from build123d import *

# Parameters (mm, degrees)
F0_R     = 2.38125
F1_DEPTH = 6.35


with BuildPart() as f1:
    # F0 (on Top) → F1 (new body)
    with BuildSketch(Plane.XY):
        with BuildLine():
            Line((77.357605, 85.293555), (-62.342395, 85.293555))
            Line((-62.342395, 85.293555), (-62.342395, 40.843555))
            Line((-62.342395, 40.843555), (-46.467395, 40.843555))
            ThreePointArc((-46.467395, 40.843555), (-41.977267, 38.983683), (-40.117395, 34.493555))
            Line((-40.117395, 34.493555), (-40.117395, -48.056445))
            ThreePointArc((-40.117395, -48.056445), (-41.977267, -52.546573), (-46.467395, -54.406445))
            Line((-46.467395, -54.406445), (-62.342395, -54.406445))
            Line((-62.342395, -54.406445), (-62.342395, -98.856445))
            Line((-62.342395, -98.856445), (-11.542395, -98.856445))
            Line((-11.542395, -98.856445), (77.357605, -98.856445))
            Line((77.357605, -98.856445), (77.357605, -54.406445))
            Line((77.357605, -54.406445), (61.482605, -54.406445))
            ThreePointArc((61.482605, -54.406445), (56.992477, -52.546573), (55.132605, -48.056445))
            Line((55.132605, -48.056445), (55.132605, 34.493555))
            ThreePointArc((55.132605, 34.493555), (56.992477, 38.983683), (61.482605, 40.843555))
            Line((61.482605, 40.843555), (77.357605, 40.843555))
            Line((77.357605, 40.843555), (77.357605, 85.293555))
        make_face()
        with Locations((-11.542395, -60.756445)):
            Circle(F0_R, mode=Mode.SUBTRACT)
        with Locations((26.557605, -60.756445)):
            Circle(F0_R, mode=Mode.SUBTRACT)
        with Locations((-40.117395, 45.606055)):
            Circle(F0_R, mode=Mode.SUBTRACT)
        with Locations((-33.767395, 40.843555)):
            Circle(F0_R, mode=Mode.SUBTRACT)
        with Locations((-40.117395, 66.243555)):
            Circle(F0_R, mode=Mode.SUBTRACT)
        with Locations((-40.117395, 80.531055)):
            Circle(F0_R, mode=Mode.SUBTRACT)
        with Locations((48.782605, 40.843555)):
            Circle(F0_R, mode=Mode.SUBTRACT)
        with Locations((55.132605, 45.606055)):
            Circle(F0_R, mode=Mode.SUBTRACT)
        with Locations((55.132605, 66.243555)):
            Circle(F0_R, mode=Mode.SUBTRACT)
        with Locations((55.132605, 80.531055)):
            Circle(F0_R, mode=Mode.SUBTRACT)
    extrude(amount=F1_DEPTH)


solid = f1.part
Model file for the job. Use its own axes, mm. A direction names the side the tool comes from. Give positions to 0.01 mm unless a question says otherwise; leave off trailing zeros. Write each loop counter-clockwise with the first axis right and the second up, starting at its lowest first coordinate (ties: lowest second). Pieces come first, ordered by that corner, then holes. Notation, with made-up numbers: (76.5, 8.25) - (98.5, 8.25) arc R18 cw to (98.5, 17.25) - close; hole circle Ø2 at (30.5, 20). An arc over 180 degrees is marked (long way). Answer as CSV lines item,"result".
1. Band-saw the part on C-C (y = -32.5). Write the cut outline in (x, z), and give its area (3 significant figures).
Responses:
outline,"(-40.12, 0) - (55.13, 0) - (55.13, 6.35) - (-40.12, 6.35) - close"
area,"605 mm2"
2. Drill centre lines: L1, parallel to Y at x = -40, z = 6.25; L2, parallel to Y at x = 54, z = 0.75; L3, parallel to Y at x = 49, z = 3.75. Where is each one in solid material? Low to high. Write a range as [from, to].
Responses:
L1,"y = [-98.86, 43.23], [47.98, 63.87], [68.62, 78.15], [82.91, 85.29]"
L2,"y = [-98.86, 43.51], [47.7, 64.15], [68.34, 78.44], [82.63, 85.29]"
L3,"y = [-98.86, 38.47], [43.21, 85.29]"
3. Two-plate mould, pull along Y, no slides. Class faces 1 (the face through (28.757, -61.668, 3.131)), 2 (the face through (77.358, -77, 3)), 3 (the face through (8, 85.294, 3)): +Y half, -Y half, draft (parallel to the pull), parting line (faces both ways), or undercut.
Responses:
face 1,"undercut"
face 2,"draft"
face 3,"+Y half"
4. 3-axis set-ups, long thin cutter, end or side, ignore diameter. For faces 4 (the face through (70, -54.406, 3)), 5 (the face through (-39.02, 64.13, 3.13)), 6 (the face through (-41.93, -52.5, 3.13)): which of +Z, -Z, +X, -X, +Y, -Y reach the whole face in a straight line?
Responses:
face 4,"+Z, -Z, +X"
face 5,"+Z, -Z"
face 6,"+Z, -Z, -X"
5. Band-saw the part on A-A (x = 66.5). Write the cut outline in (y, z).
Responses:
outline,"(-98.86, 0) - (-54.41, 0) - (-54.41, 6.35) - (-98.86, 6.35) - close; (40.84, 0) - (85.29, 0) - (85.29, 6.35) - (40.84, 6.35) - close"
6. Pin check, flat tip, straight feed: pin 1 (3 mm diameter, centred on y = 1.5, z = 3, fed in from +X). Stop position of the tip, or through.
Responses:
pin 1,"stops at x = 55.13"
7. Band-saw the part on B-B (z = 1.5). Count the separate pieces of the cut face and the enclosed holes in it, and give its area (3 significant figures).
Responses:
separate pieces,"1"
enclosed holes,"10"
area,"21,300 mm2"
